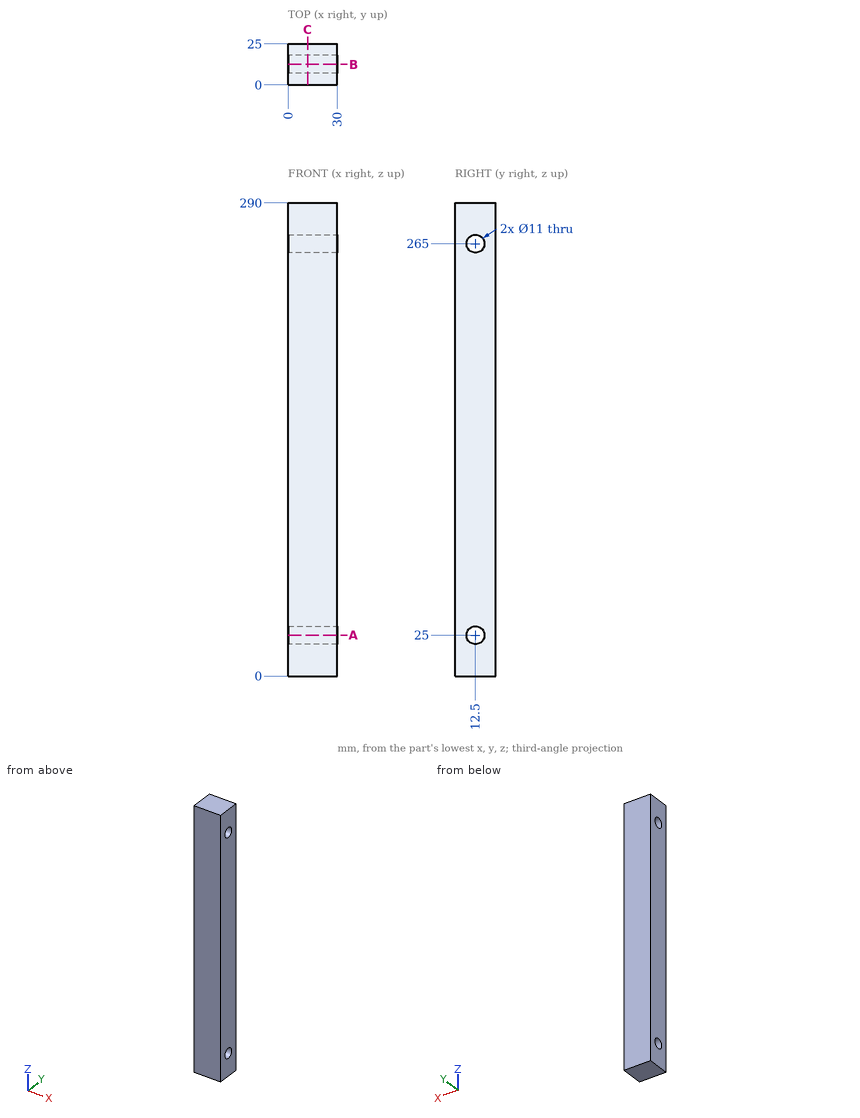
Input: dimensioned drawing with shaded views. Units: mm. Origin: part minimum x, y, z. Round coordinates to 2 decimals unless told otherwise and drop trailing zeros. Order: outer loops, then holes, each group sorted by start corner. A loop starts at its lowest first (then second) coordinate and runs counter-clockwise, first axis right, second up. Notation, with made-up numbers: M 77.5,69 L 136.5,69 A17 ccw 136.5,76 Z; hole C 38.25,-25 d10. An arc over 180 degrees is marked long. Use one line per item in the form item = value. Start each with the question number.
Q1. Cut plane A-A (z = 25). Return loops of the section in (x, y).
Q2. Cut plane B-B (y = 12.5). Return loops of the section in (x, z).
Q3. Cut plane C-C (x = 12). Return loops of the section in (y, z), and give its area (3 significant figures).
Q4. Pin query (flat end, axial travel): pin 1 Ø9 at (y, z) = (12.5, 265) entering from +X. Return the tip coordinate at first contact, or that it passes through.
Q5. Material intervals for line 1 (Y direction, x = 18.25, z = 25); line 2 (Z direction, x = 17, y = 10.5); line 3 (Z direction, x = 4.5, y = 11), sorted ascending. Write a range as [from, to].
Geometry results:
q1.outline = M 0,0 L 30,0 L 30,7 L 0,7 Z; M 0,18 L 30,18 L 30,25 L 0,25 Z
q2.outline = M 0,0 L 30,0 L 30,19.5 L 0,19.5 Z; M 0,30.5 L 30,30.5 L 30,259.5 L 0,259.5 Z; M 0,270.5 L 30,270.5 L 30,290 L 0,290 Z
q3.outline = M 0,0 L 25,0 L 25,290 L 0,290 Z; hole C 12.5,25 d11; hole C 12.5,265 d11
q3.area = 7,060 mm^2
q4.pin_1 = through
q5.line_1 = [0, 7], [18, 25]
q5.line_2 = [0, 19.88], [30.12, 259.88], [270.12, 290]
q5.line_3 = [0, 19.71], [30.29, 259.71], [270.29, 290]
